from build123d import *

# Parameters (mm, degrees)
SKETCH1_W           = 191
SKETCH1_H           = 83
BOSS_EXTRUDE2_DEPTH = 20
SKETCH3_W           = 185
SKETCH3_H           = 77
CUT_EXTRUDE2_DEPTH  = 17
SKETCH5_W           = 125
SKETCH5_H           = 21.405857205
CUT_EXTRUDE3_DEPTH  = 17


with BuildPart() as part:
    # Sketch1 → Boss-Extrude2 (new body)
    with BuildSketch(Plane(origin=(0, 0, 0), x_dir=(1, 0, 0), z_dir=(0, 1, 0))):
        Rectangle(SKETCH1_W, SKETCH1_H)
    extrude(amount=BOSS_EXTRUDE2_DEPTH)

    # Sketch3 → Cut-Extrude2 (cut)
    with BuildSketch(Plane(origin=(0, 20, 0), x_dir=(1, 0, 0), z_dir=(0, 1, 0))):
        Rectangle(SKETCH3_W, SKETCH3_H)
    extrude(amount=-CUT_EXTRUDE2_DEPTH, mode=Mode.SUBTRACT)

    # Sketch5 → Cut-Extrude3 (cut)
    with BuildSketch(Plane.XY.offset(41.5)):
        with Locations((13, 18.697690384)):
            Rectangle(SKETCH5_W, SKETCH5_H)
    extrude(amount=-CUT_EXTRUDE3_DEPTH, mode=Mode.SUBTRACT)


solid = part.part
Can you work these out from the model? Positions are in its coordinate system, mm. A direction names the side the tool comes from. Round coordinates to 2 decimals unless told otherwise and drop trailing zeros. Loops run counter-clockwise (first coordinate to the right, second up) from the corner with the lowest first, then second, coordinate; pieces in that order, holes last. Notation, with made-up numbers: (61, 28) - (76, 28) arc R20 ccw to (76, 44) - close; hole circle Ø4 at (76.25, 38). An arc over 180 degrees is marked (long way). Use CSV: the item, a comma, the result in double quotes. Start each with the question number.
1) If we section it at C-C on z = -4: Write out the boundary of the cut face in (x, y), plus the area to 3 significant figures.
2) For faces 5 (the flat face through (-1, 12, -38.5)), 6 (the flat face through (-1, 10, -41.5)), which set-ups out of +Z, -Z, +X, -X, +Y, -Y let a thin tool reach every point of the face, with its end or its side?
3) We'd pull the mould along X, two halves only. Please class faces 1 (the flat face through (-1, 0, -1)), 2 (the flat face through (-92.5, 12, 1)), 3 (the flat face through (95.5, 10, 1)), 4 (the flat face through (-1.3, 7.8, 38.5)): released by +X, released by -X, zero draft, split by the parting line, or undercut.
4) If we section it at B-B on x = -69: Write out the boundary of the cut face in (y, z).
5) If we section it at D-D on y = 14.5: Write out the boundary of the cut face in (x, z), plus the area to 3 significant figures.
6) Please list where these lines run through material, in increasing order: probe 1 along X at (y, z) = (5.5, 17); probe 2 along Z at (x, y) = (2, 4.25); probe 3 along Y at (x, z) = (-24, -8). Write a range as [from, to].
7) For pin 1 Ø1.5 at (x, z) = (-16, 40) entering from +Y; pin 2 Ø12 at (x, z) = (28.5, 1) entering from +Y, each with a flat end and sliding along its axis, tell me the tip position at first contact or that it passes through.
8) If we section it at A-A on y = 5: Write out the boundary of the cut face in (x, z), plus the area to 3 significant figures.
Geometry results:
1,outline,"(-95.5, 0) - (95.5, 0) - (95.5, 20) - (92.5, 20) - (92.5, 3) - (-92.5, 3) - (-92.5, 20) - (-95.5, 20) - close"
1,area,"675 mm2"
2,face 5,"+Y"
2,face 6,"-Z, +X, -X, +Y, -Y"
3,face 1,"zero draft"
3,face 2,"undercut"
3,face 3,"released by +X"
3,face 4,"undercut"
4,outline,"(0, -41.5) - (20, -41.5) - (20, -38.5) - (3, -38.5) - (3, 38.5) - (20, 38.5) - (20, 41.5) - (0, 41.5) - close"
5,outline,"(-95.5, -41.5) - (95.5, -41.5) - (95.5, 41.5) - (75.5, 41.5) - (75.5, 38.5) - (92.5, 38.5) - (92.5, -38.5) - (-92.5, -38.5) - (-92.5, 38.5) - (-49.5, 38.5) - (-49.5, 41.5) - (-95.5, 41.5) - close"
5,area,"1,230 mm2"
6,probe 1,"x = [-95.5, -92.5], [92.5, 95.5]"
6,probe 2,"z = [-41.5, -38.5], [38.5, 41.5]"
6,probe 3,"y = [0, 3]"
7,pin 1,"stops at y = 7.99"
7,pin 2,"stops at y = 3"
8,outline,"(-95.5, -41.5) - (95.5, -41.5) - (95.5, 41.5) - (-95.5, 41.5) - close; hole (-92.5, -38.5) - (92.5, -38.5) - (92.5, 38.5) - (-92.5, 38.5) - close"
8,area,"1,610 mm2"
